```python
from build123d import *

# Parameters (mm, degrees)
SKETCH_1_W             = 195
SKETCH_1_H             = 16
EXTRUDE_1_DEPTH        = 25
EXTRUDE_2_DEPTH        = 25
PATTERN_LINEAR_1_COUNT = 10
PATTERN_LINEAR_1_PITCH = 8
PATTERN_LINEAR_2_COUNT = 10
PATTERN_LINEAR_2_PITCH = 8
SKETCH_3_W             = 195
SKETCH_3_H             = 4
EXTRUDE_3_DEPTH        = 5
SKETCH_5_W             = 195
SKETCH_5_H             = 4
EXTRUDE_4_DEPTH        = 5
SKETCH_6_W             = 20
SKETCH_6_H             = 25
EXTRUDE_5_DEPTH        = 7
EXTRUDE_6_DEPTH        = 7
EXTRUDE_START          = -7
EXTRUDE_7_DEPTH        = 7
SKETCH_9_R             = 4.5
CUT_EXTRUDE_1_DEPTH    = 50
SKETCH_10_R            = 4.5
CUT_EXTRUDE_2_DEPTH    = 50


with BuildPart() as part:
    # Sketch 1 → Extrude 1 (new body)
    with BuildSketch(Plane.XY):
        Rectangle(SKETCH_1_W, SKETCH_1_H)
    extrude(amount=EXTRUDE_1_DEPTH)

    # Sketch 2 → Extrude 2 (add)
    with BuildSketch(Plane.XY.offset(25)):
        with BuildLine():
            Line((-2.5, 8), (2.5, 8))
            add(Edge.make_bspline(
                [(2.5, 8), (2.5, 9.044984292), (1.579923026, 13.044978727), (1.25, 14)],
                knots=[0, 0, 0, 0, 0.806888018, 0.806888018, 0.806888018, 0.806888018], degree=3))
            Line((1.25, 14), (-1.25, 14))
            add(Edge.make_bspline(
                [(-2.5, 8), (-2.5, 9.044984292), (-1.579923026, 13.044978727), (-1.25, 14)],
                knots=[0, 0, 0, 0, 0.806888018, 0.806888018, 0.806888018, 0.806888018], degree=3))
        make_face()
    extrude_2 = extrude(amount=-EXTRUDE_2_DEPTH)

    # Pattern Linear 1: Extrude 2 ×10
    with Locations(*[(-i * PATTERN_LINEAR_1_PITCH, 0, 0) for i in range(1, PATTERN_LINEAR_1_COUNT)]):
        add(extrude_2)

    # Pattern Linear 2: Extrude 2 ×10
    with Locations(*[(i * PATTERN_LINEAR_2_PITCH, 0, 0) for i in range(1, PATTERN_LINEAR_2_COUNT)]):
        add(extrude_2)

    # Sketch 3 → Extrude 3 (add)
    with BuildSketch(Plane.XY.offset(25)):
        with Locations((0, -6)):
            Rectangle(SKETCH_3_W, SKETCH_3_H)
    extrude(amount=EXTRUDE_3_DEPTH)

    # Sketch 5 → Extrude 4 (add)
    with BuildSketch(Plane(origin=(0, 0, 0), x_dir=(-1, 0, 0), z_dir=(0, 0, -1))):
        with Locations((0, -6)):
            Rectangle(SKETCH_5_W, SKETCH_5_H)
    extrude(amount=EXTRUDE_4_DEPTH)

    # Sketch 6 → Extrude 5 (add)
    with BuildSketch(Plane(origin=(0, 8, 0), x_dir=(1, 0, 0), z_dir=(0, 1, 0))):
        with Locations((87.5, -12.5)):
            Rectangle(SKETCH_6_W, SKETCH_6_H)
    extrude_5 = extrude(amount=EXTRUDE_5_DEPTH)

    # Sketch 7 → Extrude 6 (add)
    with BuildSketch(Plane(origin=(0, 15, 0), x_dir=(1, 0, 0), z_dir=(0, 1, 0))):
        with BuildLine():
            Line((97.5, 0), (109.5, 0))
            ThreePointArc((109.5, 0), (122, -12.5), (109.5, -25))
            Line((109.5, -25), (97.5, -25))
            Line((97.5, -25), (97.5, 0))
        make_face()
    extrude_6 = extrude(amount=-EXTRUDE_6_DEPTH)

    # Mirror 1: Extrude 5, Extrude 6 across plane
    add(extrude_5.mirror(Plane(origin=(0, 0, 0), x_dir=(0, 0, 1), z_dir=(1, 0, 0))))
    add(extrude_6.mirror(Plane(origin=(0, 0, 0), x_dir=(0, 0, 1), z_dir=(1, 0, 0))))

    # Sketch 8 → Extrude 7 (add)
    with BuildSketch(Plane.XZ.offset(8).offset(EXTRUDE_START)):
        with BuildLine():
            Line((97.5, 25), (97.5, 0))
            Line((97.5, 0), (109.5, 0))
            ThreePointArc((109.5, 0), (122, 12.5), (109.5, 25))
            Line((109.5, 25), (97.5, 25))
        make_face()
    extrude_7 = extrude(amount=EXTRUDE_7_DEPTH)

    # Mirror 2: Extrude 7 across plane
    add(extrude_7.mirror(Plane(origin=(0, 0, 0), x_dir=(0, 0, 1), z_dir=(1, 0, 0))))

    # Sketch 9 → Cut-Extrude 1 (cut)
    with BuildSketch(Plane(origin=(0, 15, 0), x_dir=(1, 0, 0), z_dir=(0, 1, 0))):
        with Locations(Location((-109.5, -12.5, 0), (0, 0, 270))):
            Circle(SKETCH_9_R)
    extrude(amount=-CUT_EXTRUDE_1_DEPTH, mode=Mode.SUBTRACT)

    # Sketch 10 → Cut-Extrude 2 (cut)
    with BuildSketch(Plane(origin=(0, 15, 0), x_dir=(1, 0, 0), z_dir=(0, 1, 0))):
        with Locations(Location((109.5, -12.5, 0), (0, 0, 270))):
            Circle(SKETCH_10_R)
    extrude(amount=-CUT_EXTRUDE_2_DEPTH, mode=Mode.SUBTRACT)


solid = part.part
```
Here's how the part is built. I have some questions about the finished solid (model axes, mm). A direction names the side the tool comes from. Coordinates: 2 decimals unless noted, no trailing zeros. Loops run counter-clockwise (first coordinate to the right, second up) from the corner with the lowest first, then second, coordinate; pieces in that order, holes last. Notation, with made-up numbers: M 65.5,-37 L 101.5,-37 A16 ccw 101.5,-13 Z; hole C 37,-10 d8. An arc over 180 degrees is marked long. One line per item, written item: value.
1. Thinking about a two-plate mould opening in X: for faces 4 (the flat face through (-77.5, 11, 13)), 5 (the flat face through (97.5, -6, -2)), 6 (the flat face through (-97.5, -6, -2)), 7 (the flat face through (-1, -6, 30)), which applies, +X half, -X half, draft (parallel to the pull), parting line (faces both ways), or undercut?
Geometry says:
face 4: undercut
face 5: +X half
face 6: -X half
face 7: draft
2. On a 3-axis mill with a long thin cutter (end or side, diameter ignored), from which of +Z, -Z, +X, -X, +Y, -Y can I reach the whole of each face in a straight line? I mean faces 1 (the flat face through (-104, 8, 12)), 2 (the flat face through (97.5, -6, 28)), 3 (the flat face through (104, -1, 13)). Say none if no direction works.
Geometry says:
face 1: +Z, -Z, -X
face 2: +Z, +X, +Y, -Y
face 3: +Z, -Z, +X
3. Will these pins go through, and if not, where does the flat tip stop? pin 1 Ø12 at (y, z) = (-1.5, 26.5) entering from -X; pin 2 Ø1.2 at (x, z) = (48.5, 8.5) entering from +Y; pin 3 Ø4 at (x, z) = (19, -3.5) entering from +Y.
Geometry says:
pin 1: stops at x = -119.1
pin 2: stops at y = 14
pin 3: stops at y = -4
4. Please list where these lines run through material, in increasing order: probe 1 along X at (y, z) = (-6, 12.5); probe 2 along Y at (x, z) = (-33, 4.5); probe 3 along Z at (x, y) = (-18.5, 7).
Geometry says:
probe 1: x = -122 to -114, -105 to 105, 114 to 122
probe 2: y = -8 to 14
probe 3: z = 0 to 25
5. Imagine slicing it at B-B (y = 3.75). List the corners of the cut face in (x, z) for me.
Geometry says:
outline: M -97.5,0 L 97.5,0 L 97.5,25 L -97.5,25 Z
6. Imagine slicing it at A-A (x = -102). List the corners of the cut face in (y, z) for me, and give its area (3 significant figures).
Geometry says:
outline: M -8,0 L -1,0 L -1,25 L -8,25 Z; M 8,0 L 15,0 L 15,25 L 8,25 Z
area: 350 mm2
